Autodesk Inventor part; units mm, degrees
ref_plane "YZ Plane" through (0, 0, 0) normal (1, 0, 0) x (0, 1, 0)
ref_plane "XZ Plane" through (0, 0, 0) normal (0, 1, 0) x (-1, 0, 0)
ref_plane "XY Plane" through (0, 0, 0) normal (0, 0, 1) x (1, 0, 0)
sketch "Эскиз1" plane through (0, 0, 0) normal (1, 0, 0) x (0, 1, 0)
  line L0 (-7.5, 25) -> (7.5, 25)
  line L1 (7.5, 25) -> (7.5, -25)
  line L2 (7.5, -25) -> (-7.5, -25)
  line L3 (-7.5, -25) -> (-7.5, 25)
  line L4 (-7.5, 25) -> (7.5, -25) construction
  line L5 (7.5, 25) -> (-7.5, -25) construction
  line L6 (0, -25) -> (0, -32.5)
  arc A0 (-7.5, -32.5) -> (7.5, -32.5) centre (0, -32.5) ccw
  line L7 (-7.5, -25) -> (-7.5, -32.5)
  line L8 (7.5, -25) -> (7.5, -32.5)
  circle A1 centre (0, -32.5) radius 2.1
  line L9 (-7.5, -32.5) -> (-7.5, -44.5)
  line L10 (-7.5, -44.5) -> (7.5, -44.5)
  line L11 (7.5, -44.5) -> (7.5, -32.5)
  line L12 (7.5, -32.5) -> (2.1, -32.5)
  line L13 (-2.1, -32.5) -> (-7.5, -32.5)
  line L14 (7.5, -44.5) -> (-7.5, -44.5)
  line L15 (-7.5, -44.5) -> (-7.5, -52.5)
  line L16 (-7.5, -52.5) -> (7.5, -52.5)
  line L17 (7.5, -52.5) -> (7.5, -44.5)
  point P0 (0, 0)
  dimension "d0" = 15
  dimension "d1" = 50
  dimension "d4" = 4.2
  dimension "d31" = 15
  dimension "d32" = 12
  dimension "d34" = 8
extrude "Выдавливание1" add sketch "Эскиз1" along normal blind 25 contours L0 L1 L2 L3 | L2 L6 A1 L13 L7 | L8 L12 A1 L6 L2 | L13 A1 L12 A0 | A0 L11 L10 L9 | L10 L17 L16 L15
sketch "Эскиз2" plane through (0, 7.5, 25) normal (0, 1, 0) x (1, 0, 0)
  line L0 (0, 65) -> (25, 65)
  line L1 (3.5, 50) -> (21.5, 50)
  line L2 (21.5, 50) -> (21.5, 65)
  line L3 (21.5, 65) -> (3.5, 65)
  line L4 (3.5, 65) -> (3.5, 50)
  line L5 (0, 57.5) -> (25, 57.5)
  line L6 (3.5, 50) -> (21.5, 65) construction
  line L7 (21.5, 50) -> (3.5, 65) construction
  point P0 (0, 25)
  point P1 (12.5, 57.5)
  dimension "d7" = 18
extrude "Выдавливание2" cut sketch "Эскиз2" against normal blind 25
sketch "Эскиз3" plane through (0, 7.5, 25) normal (0, 1, 0) x (1, 0, 0)
  line L0 (21.5, 50) -> (3.5, 50)
  line L1 (12.5, 50) -> (12.5, 35)
  line L2 (9.5, 27.5) -> (15.5, 27.5)
  line L3 (15.5, 27.5) -> (15.5, 42.5)
  line L4 (15.5, 42.5) -> (9.5, 42.5)
  line L5 (9.5, 42.5) -> (9.5, 27.5)
  line L6 (9.5, 27.5) -> (15.5, 42.5) construction
  line L7 (15.5, 27.5) -> (9.5, 42.5) construction
  point P0 (0, 25)
  dimension "d10" = 15
  dimension "d11" = 6
  dimension "d12" = 15
extrude "Выдавливание3" cut sketch "Эскиз3" against normal blind 25
sketch "Эскиз4" plane through (25, 0, 0) normal (1, 0, 0) x (0, 0, -1)
  line L0 (2.5, 7.5) -> (2.5, -7.5)
  line L1 (17.5, 7.5) -> (17.5, -7.5)
  line L2 (2.5, 7.5) -> (2.5, -7.5)
  line L3 (2.5, 0) -> (17.5, 0)
  circle A0 centre (10, 0) radius 1.8
  point P0 (0, 0)
  dimension "d15" = 3.6
extrude "Выдавливание4" cut sketch "Эскиз4" against normal blind 25
sketch "Эскиз5" plane through (25, 0, 0) normal (1, 0, 0) x (0, 0, -1)
  circle A0 centre (10, 0) radius 1.8
  circle A1 centre (10, 0) radius 5
  point P0 (0, 0)
  dimension "d18" = 10
extrude "Выдавливание5" cut sketch "Эскиз5" against normal blind 5
fillet "Сопряжение1" radius 7.5 2 edges at (12.5, 7.5, 25) (12.5, -7.5, 25)
sketch "Эскиз6" plane through (25, 0, 0) normal (1, 0, 0) x (0, 0, -1)
  arc A0 (-17.5, 7.5) -> (-17.5, -7.5) centre (-17.5, 0) ccw
  circle A1 centre (-17.5, 0) radius 2.85
  point P0 (0, 0)
  dimension "d22" = 5.7
extrude "Выдавливание6" cut sketch "Эскиз6" against normal blind 25
sketch "Эскиз7" plane through (3.5, 7.5, -25) normal (0, 1, 0) x (1, 0, 0)
  line L0 (-3.5, -50) -> (21.5, -50)
  line L1 (0, -35) -> (18, -35)
  line L2 (18, -35) -> (18, -50)
  line L3 (18, -50) -> (0, -50)
  line L4 (0, -50) -> (0, -35)
  line L5 (-3.5, -42.5) -> (21.5, -42.5)
  line L6 (0, -35) -> (18, -50) construction
  line L7 (18, -35) -> (0, -50) construction
  point P0 (-3.5, -25)
  point P1 (9, -42.5)
  dimension "d25" = 18
extrude "Выдавливание7" cut sketch "Эскиз7" against normal blind 25
chamfer "Фаска1" distance 3.25 angle 45 4 edges at (12.5, 7.5, 10) (12.5, -7.5, 10) (12.5, 7.5, -25) (12.5, -7.5, -25)
fillet "Сопряжение3" radius 7.5 2 edges at (12.5, 7.5, -52.5) (12.5, -7.5, -52.5)
sketch "Эскиз8" plane through (25, 0, 0) normal (1, 0, 0) x (0, 0, -1)
  circle A0 centre (48.2471, 0) radius 2
  point P0 (0, 0)
  dimension "d36" = 4
extrude "Выдавливание8" cut sketch "Эскиз8" against normal blind 25
sketch "Эскиз9" plane through (0, 7.5, 17.5) normal (0, 1, 0) x (1, 0, 0)
  line L0 (25, 62.5) -> (0, 62.5)
  line L1 (0, 70) -> (25, 70)
  line L2 (8.611, 62.5) -> (15.9557, 62.5)
  line L3 (15.9557, 62.5) -> (15.9557, 70)
  line L4 (15.9557, 70) -> (8.611, 70)
  line L5 (8.611, 70) -> (8.611, 62.5)
  point P0 (0, 17.5)
extrude "Выдавливание9" cut sketch "Эскиз9" against normal blind 25
properties part number "КВ33.044.602 - Держатель катка"
Part model, mm, in its own coordinate system. A direction names the side the tool comes from. Coordinates: 2 decimals unless noted, no trailing zeros. Loops run counter-clockwise (first coordinate to the right, second up) from the corner with the lowest first, then second, coordinate; pieces in that order, holes last. Notation, with made-up numbers: (-31.5, 49) - (8.5, 49) arc R21 ccw to (8.5, 84) - close; hole circle Ø6 at (10.25, 8.25). An arc over 180 degrees is marked (long way). Write item = value, one per line. Start each with the question number.
Item 1: Cut at A-A, the plane z = -32.5. Give the cut face in (x, y).
Item 2: 3-axis set-ups, long thin cutter, end or side, ignore diameter. For faces 1 (the flat face through (12.63, 5.85, -23.4)), 2 (the flat face through (12, 0, -2.5)), 3 (the flat face through (12.37, -5.85, -23.4)), 4 (the flat face through (15.956, 0, -46)): which of +Z, -Z, +X, -X, +Y, -Y reach the whole face in a straight line?
Item 3: Mould opens along Y. For faces 5 (the flat face through (12.63, 5.85, 8.4)), 6 (the flat face through (20, -2, -10)), 7 (the flat face through (25, -5, -13)), 8 (the cylindrical face through (22.54, 1.5, -14.77)) say: released by +Y, released by -Y, zero draft, split by the parting line, or undercut.
Item 4: Cut at C-C, the plane z = -16. Give the cut face in (x, y).
Item 5: Cut at D-D, the plane x = 2. State how many separate pieces and enclosed holes the cut face has, and give its area (3 significant figures).
Item 6: Cut at B-B, the plane x = 13.5. Give the cut face in (y, z).
Item 7: Flat gauge pins, fed straight in: pin 1 Ø6 at (x, y) = (13.5, 2.5) entering from -Z; pin 2 Ø3 at (x, y) = (14, 0.5) entering from +Z; pin 3 Ø6 at (y, z) = (0, -10) entering from +X. Where does each tip first touch, or does it go through?
Item 8: Wall check: L1, parallel to Z at x = 14.5, y = -3.5; L2, parallel to X at y = 0.5, z = -27; L3, parallel to X at y = 0, z = -3. Give the ranges that are in metal, low to high. Write a range as from..to.
The answers:
q1.outline = (0, -7.5) - (3.5, -7.5) - (3.5, -2.1) - (0, -2.1) - close; (0, 2.1) - (3.5, 2.1) - (3.5, 7.5) - (0, 7.5) - close; (21.5, -7.5) - (25, -7.5) - (25, -2.1) - (21.5, -2.1) - close; (21.5, 2.1) - (25, 2.1) - (25, 7.5) - (21.5, 7.5) - close
q2.face_1 = +Y
q2.face_2 = +Y, -Y
q2.face_3 = -Y
q2.face_4 = -Z, +Y, -Y
q3.face_5 = released by +Y
q3.face_6 = undercut
q3.face_7 = zero draft
q3.face_8 = undercut
q4.outline = (0, -7.5) - (9.5, -7.5) - (9.5, 7.5) - (0, 7.5) - close; (15.5, -7.5) - (25, -7.5) - (25, 7.5) - (15.5, 7.5) - close
q5.separate_pieces = 1
q5.enclosed_holes = 4
q5.area = 1,050 mm2
q6.outline = (-7.5, -45) - (7.5, -45) - (7.5, -40) - (-7.5, -40) - close; (-7.5, -21.75) - (-4.25, -25) - (4.25, -25) - (7.5, -21.75) - (7.5, -17.5) - (-7.5, -17.5) - close; (-7.5, -2.5) - (7.5, -2.5) - (7.5, 6.75) - (4.25, 10) - (-4.25, 10) - (-7.5, 6.75) - close
q7.pin_1 = -52.46
q7.pin_2 = 10
q7.pin_3 = 20
q8.L1 = -45..-40, -25..-17.5, -2.5..10
q8.L2 = 0..3.5, 21.5..25
q8.L3 = 0..9.5, 15.5..25
